```python
from build123d import *

# Parameters (mm, degrees)
SKETCH_1_W                       = 50
SKETCH_1_H                       = 23
CUT_EXTRUDE_1_DEPTH              = 109.388191239
FILLET_1_R                       = 2
PATTERN_CIRCULAR_1_COUNT         = 6
FILLET_1_OF_PATTERN_CIRCULAR_1_R = 2


with BuildPart() as part:
    # Эскиз1 → Повернуть1 (revolve)
    with BuildSketch(Plane(origin=(0, 0, 0), x_dir=(0, 0, -1), z_dir=(1, 0, 0)), mode=Mode.PRIVATE) as revolve_1_sk:
        with Locations((25, 56.5)):
            Rectangle(SKETCH_1_W, SKETCH_1_H)
    revolve(revolve_1_sk.sketch.rotate(Axis((0, 0, 0), (0, 0, -1)), 90), axis=Axis((0, 0, 0), (0, 0, -1)))

    # Эскиз2 → Вырез-Вытянуть1 (cut, through all)
    with BuildSketch(Plane.XY):
        with BuildLine():
            Line((-8.8, 59.351158371), (-8.8, 44.131168124))
            ThreePointArc((-8.8, 44.131168124), (-15.861240947, 42.112005837), (-22.5, 38.97114317))
            Line((-22.5, 38.97114317), (-30, 51.961524227))
            ThreePointArc((-30, 51.961524227), (-19.748713204, 56.65675888), (-8.8, 59.351158371))
        make_face()
        with BuildLine():
            Line((8.8, 59.351158371), (8.8, 44.131168124))
            ThreePointArc((8.8, 44.131168124), (15.861240947, 42.112005837), (22.5, 38.97114317))
            Line((22.5, 38.97114317), (30, 51.961524227))
            ThreePointArc((30, 51.961524227), (19.748713204, 56.65675888), (8.8, 59.351158371))
        make_face()
    cut_extrude_1 = extrude(amount=-CUT_EXTRUDE_1_DEPTH, mode=Mode.SUBTRACT)

    # Скругление1
    fillet_1_edges = [part.edges().sort_by_distance(p)[0] for p in [
        (-8.8, 59.351158371, -25),
        (8.8, 59.351158371, -25),
    ]]
    fillet(fillet_1_edges, radius=FILLET_1_R)

    # Круговой массив1: Вырез-Вытянуть1 ×6 about axis
    pattern_circular_1_axis = Axis((0, 0, 0), (0, 0, 1))
    for i in range(1, PATTERN_CIRCULAR_1_COUNT):
        add(cut_extrude_1.rotate(pattern_circular_1_axis, i * 360 / PATTERN_CIRCULAR_1_COUNT), mode=Mode.SUBTRACT)

    # Скругление1 of Круговой массив1
    fillet_1_of_pattern_circular_1_edges = [part.edges().sort_by_distance(p)[0] for p in [
        (-55.799610893, 22.054555632, -25),
        (-46.999610893, 37.296602739, -25),
        (-46.999610893, -37.296602739, -25),
        (-55.799610893, -22.054555632, -25),
        (8.8, -59.351158371, -25),
        (-8.8, -59.351158371, -25),
        (55.799610893, -22.054555632, -25),
        (46.999610893, -37.296602739, -25),
        (46.999610893, 37.296602739, -25),
        (55.799610893, 22.054555632, -25),
    ]]
    fillet(fillet_1_of_pattern_circular_1_edges, radius=FILLET_1_OF_PATTERN_CIRCULAR_1_R)


solid = part.part
```
Could you check a few things on this model? Use its own coordinates, in mm. Coordinates: 2 decimals unless noted, no trailing zeros. Loops run counter-clockwise (first coordinate to the right, second up) from the corner with the lowest first, then second, coordinate; pieces in that order, holes last. Notation, with made-up numbers: M 83,84 L 122,84 A29 ccw 122,117 Z; hole C -6,70 d8. An arc over 180 degrees is marked long. Put each result on its own line as item: value. Start each with the question number.
(1) I need wall thicknesses on line 1 (X direction, y = 52, z = -5); line 2 (X direction, y = 54, z = -13); line 3 (X direction, y = -33.5, z = -5.5). Which ranges of each line are inside material? Lowest first, please. Write a range as from..to.
(2) Thinking about a two-plate mould opening in Y: for faces 1 (the face through (41, -20, 0)), 2 (the face through (-45.927, 37.535, -25.35)), which applies, pulls with the +Y half, pulls with the -Y half, needs draft (parallel to the pull), parting line crosses it, or undercut?
(3) Suppose I cut it at D-D on x = 22.5. Please give me the cut outline in (y, z), then the cut area to 3 significant figures.
(4) Suppose I cut it at C-C on x = 39.5. Please give me the cut outline in (y, z).
(5) Suppose I cut it at B-B on y = 54. Please give me the cut outline in (x, z).
(6) Will these pins go through, and if not, where does the flat tip stop? P1, Ø14, axis at y = -51.5, z = -36, coming from the -X side; P2, Ø4, axis at x = -22, z = -34, coming from the -Y side; P3, Ø10, axis at y = -21.5, z = -43, coming from the -X side.
(7) Suppose I cut it at A-A on x = 0. Please give me the cut outline in (y, z), then the cut area to 3 significant figures.
Solutions:
1. line 1: x = -43.82..-29.93, -8.8..8.8, 29.93..43.82
1. line 2: x = -41.33..-26.15, -8.8..8.8, 26.15..41.33
1. line 3: x = -59.18..-40.42, 40.42..59.18
2. face 1: needs draft
2. face 2: undercut
3. outline: M -64.17,-50 L -55.62,-50 L -55.62,0 L -64.17,0 Z; M 55.62,-50 L 64.17,-50 L 64.17,0 L 55.62,0 Z
3. area: 855 mm2
4. outline: M -55.35,-50 L -45.16,-50 L -45.16,0 L -55.35,0 Z; M -32.97,-50 L -21.56,-50 L -21.56,0 L -32.97,0 Z; M 21.56,-50 L 32.97,-50 L 32.97,0 L 21.56,0 Z; M 45.16,-50 L 55.35,-50 L 55.35,0 L 45.16,0 Z
5. outline: M -41.33,-50 L -26.15,-50 L -26.15,0 L -41.33,0 Z; M -8.8,-50 L 8.8,-50 L 8.8,0 L -8.8,0 Z; M 26.15,-50 L 41.33,-50 L 41.33,0 L 26.15,0 Z
6. P1: stops at x = -51.42
6. P2: stops at y = -64.99
6. P3: stops at x = -65.97
7. outline: M -68,-50 L -45,-50 L -45,0 L -68,0 Z; M 45,-50 L 68,-50 L 68,0 L 45,0 Z
7. area: 2,300 mm2
